Input: part model. Units: mm. Frame: model coordinates. A direction names the side the tool comes from. Round coordinates to 2 decimals unless told otherwise and drop trailing zeros. Loops run counter-clockwise (first coordinate to the right, second up) from the corner with the lowest first, then second, coordinate; pieces in that order, holes last. Notation, with made-up numbers: (35.25, 56) - (87.25, 56) arc R15 ccw to (87.25, 84) - close; hole circle Ø1 at (-35.5, 54). An arc over 180 degrees is marked (long way). One line per question, with ' | ' between items. Start each with the question number.
Item 1: Draft query along Y for faces 6 (the face through (6, -19, 5.466)), 7 (the face through (6, -38.1, 3)), 8 (the face through (4, -8.687, 3)), 9 (the face through (3, 0, 3)). Return one class per face: pulls with the +Y half, pulls with the -Y half, needs draft (parallel to the pull), parting line crosses it, or undercut.
Item 2: Section C-C, the plane z = 2.35. Return loops of the section in (x, y).
Item 3: Section B-B, the plane y = -3. Return loops of the section in (x, z).
Item 4: Section D-D, the plane x = 5. Return loops of the section in (y, z).
Item 5: First-contact query: pin 1 (3 mm diameter, centred on y = -7, z = 1.5, fed in from -X). Flat tip, straight axial feed; report the tip coordinate or a pass-through.
Item 6: Section A-A, the plane x = 10.25. Return loops of the section in (y, z), plus the area to 3 significant figures.
Item 7: Material intervals for line 1 along Y through (x, z) = (5.5, 3.65); line 2 along Y through (x, z) = (9.5, 2.05); line 3 along X through (y, z) = (-10, 1.3), sorted ascending.
Item 8: Set-up query: faces 1 (the face through (6, -19, 0)), 2 (the face through (6.248, -31, 3)), 3 (the face through (2, -34.773, 3)), 4 (the face through (5.639, -3, 3)), 5 (the face through (10, 0, 3)). Return all of +Z, -Z, +X, -X, +Y, -Y with unobstructed straight access to the full face (end or side cutting, diameter ignored); none if empty.
```python
from build123d import *

# Parameters (mm, degrees)
F0_W     = 12.3952
F0_H     = 5.465724
F1_DEPTH = 38.1
F3_DEPTH = 25.4
F4_DEPTH = 25.4


with BuildPart() as f1:
    # F0 (on Front) → F1 (new body)
    with BuildSketch(Plane.XZ):
        with Locations((6.1976, 2.732862)):
            Rectangle(F0_W, F0_H)
    extrude(amount=F1_DEPTH)

    # F2 (on face) → F3 (cut)
    with BuildSketch(Plane.XY.offset(5.465724)):
        Polygon((8.179207, 0), (5.639207, 0), (5.639207, -6.1468), (3.099207, -6.1468), (3.099207, -8.6868), (5.639207, -8.6868), (5.639207, -11.2268), (8.179207, -11.2268), (8.179207, -8.6868), (10.719207, -8.6868), (10.719207, -6.1468), (8.179207, -6.1468), align=None)
    extrude(amount=-F3_DEPTH, mode=Mode.SUBTRACT)

    # F2 (on face) → F4 (cut)
    with BuildSketch(Plane.XY.offset(5.465724)):
        Polygon((12.3952, -34.77345), (12.3952, -32.23345), (6.2484, -32.23345), (6.2484, -29.69345), (3.7084, -29.69345), (3.7084, -32.23345), (1.1684, -32.23345), (1.1684, -34.77345), (3.7084, -34.77345), (3.7084, -37.31345), (6.2484, -37.31345), (6.2484, -34.77345), align=None)
    extrude(amount=-F4_DEPTH, mode=Mode.SUBTRACT)


solid = f1.part
```
Return value:
1) face 6: needs draft | face 7: pulls with the -Y half | face 8: undercut | face 9: pulls with the +Y half
2) outline: (0, -38.1) - (12.4, -38.1) - (12.4, -34.77) - (6.25, -34.77) - (6.25, -37.31) - (3.71, -37.31) - (3.71, -34.77) - (1.17, -34.77) - (1.17, -32.23) - (3.71, -32.23) - (3.71, -29.69) - (6.25, -29.69) - (6.25, -32.23) - (12.4, -32.23) - (12.4, 0) - (8.18, 0) - (8.18, -6.15) - (10.72, -6.15) - (10.72, -8.69) - (8.18, -8.69) - (8.18, -11.23) - (5.64, -11.23) - (5.64, -8.69) - (3.1, -8.69) - (3.1, -6.15) - (5.64, -6.15) - (5.64, 0) - (0, 0) - close
3) outline: (0, 0) - (5.64, 0) - (5.64, 5.47) - (0, 5.47) - close; (8.18, 0) - (12.4, 0) - (12.4, 5.47) - (8.18, 5.47) - close
4) outline: (-38.1, 0) - (-37.31, 0) - (-37.31, 5.47) - (-38.1, 5.47) - close; (-29.69, 0) - (-8.69, 0) - (-8.69, 5.47) - (-29.69, 5.47) - close; (-6.15, 0) - (0, 0) - (0, 5.47) - (-6.15, 5.47) - close
5) pin 1: x = 0
6) outline: (-38.1, 0) - (-34.77, 0) - (-34.77, 5.47) - (-38.1, 5.47) - close; (-32.23, 0) - (-8.69, 0) - (-8.69, 5.47) - (-32.23, 5.47) - close; (-6.15, 0) - (0, 0) - (0, 5.47) - (-6.15, 5.47) - close | area: 180 mm2
7) line 1: -38.1 to -37.31, -29.69 to -8.69, -6.15 to 0 | line 2: -38.1 to -34.77, -32.23 to -8.69, -6.15 to 0 | line 3: 0 to 5.64, 8.18 to 12.4
8) face 1: -Z, +X, -X, +Y, -Y | face 2: +Z, -Z | face 3: +Z, -Z, +X | face 4: +Z, -Z, +Y | face 5: +Z, -Z, +X, -X, +Y
